The model under review builds one solid part; all positions refer to its coordinate system, in mm. A direction names the side the tool comes from. Coordinates: 2 decimals unless noted, no trailing zeros. Loops run counter-clockwise (first coordinate to the right, second up) from the corner with the lowest first, then second, coordinate; pieces in that order, holes last. Notation, with made-up numbers: M 59.25,-17 L 78.25,-17 A22 ccw 78.25,13 Z; hole C 16.25,36 d4. An arc over 180 degrees is marked long. Use CSV: the item, a comma, the result in double quotes. Start each with the question number.
1. Add section B-B, the plane x = 5.5. Write out the cut boundary in (y, z).
2. Add section A-A, the plane y = 3.5. Write out the cut boundary in (x, z).
3. Add section D-D, the plane x = 2.25. Write out the cut boundary in (y, z), then the cut area to 3 significant figures.
4. Add section C-C, the plane z = 0.25. Write out the cut boundary in (x, y).
5. Tool access review of faces 1 (the cylindrical face through (1.479, -3.859, 2.797)), 2 (the flat face through (0, 0, 0)), 3 (the flat face through (5.2, -2.5, -3)), 4 (the flat face through (5.2, -3, -3.5)), 5 (the flat face through (4, 4, 2)): name each direction out of +Z, -Z, +X, -X, +Y, -Y from which nothing blocks a thin tool from reaching the whole face with its end or side.
6. For L1, parallel to Z at x = 6.25, y = 2.5; L2, parallel to Z at x = 4.75, y = 3.5; L3, parallel to X at y = 1.5, z = 2, list the stretches that pass through material, from the lowest coordinate up.
7. Clearance check with flat-ended pins moving along their axes: P1, Ø1.3, axis at x = 6, y = 2, coming from the +Z side; P2, Ø1.1, axis at x = 6, y = -2.5, coming from the +Z side; P3, Ø1, axis at y = 3, z = 1, coming from the +X side. State where each tip first meets the part, or that it passes through.
from build123d import *

# Parameters (mm, degrees)
BOSS_EXTRUDE1_DEPTH = 3
BOSS_EXTRUDE2_DEPTH = 4.5
BOSS_EXTRUDE3_DEPTH = 3


with BuildPart() as part:
    # Sketch1 → Boss-Extrude1 (new body)
    with BuildSketch(Plane(origin=(0, 0, 0), x_dir=(0, 0, -1), z_dir=(1, 0, 0))):
        with BuildLine():
            Line((4, -5), (0, -5))
            ThreePointArc((0, -5), (-2.828427125, -3.828427125), (-4, -1))
            Line((-4, -1), (-4, 5))
            Line((-4, 5), (4, 5))
            Line((4, 5), (4, -5))
        make_face()
    extrude(amount=BOSS_EXTRUDE1_DEPTH)

    # Sketch2 → Boss-Extrude2 (add)
    with BuildSketch(Plane(origin=(3, 0, 0), x_dir=(0, 0, -1), z_dir=(1, 0, 0))):
        Polygon((4, -3), (4, 5), (2, 5), (2, -2), (3, -2), (3, -3), align=None)
    extrude(amount=BOSS_EXTRUDE2_DEPTH)

    # Sketch3 → Boss-Extrude3 (add)
    with BuildSketch(Plane(origin=(3, 0, 0), x_dir=(0, 0, -1), z_dir=(1, 0, 0))):
        with BuildLine():
            Line((2, 0), (2, 5))
            Line((2, 5), (-2, 5))
            Line((-2, 5), (-2, 3))
            ThreePointArc((-2, 3), (0.121320344, 2.121320344), (1, 0))
            Line((1, 0), (2, 0))
        make_face()
    extrude(amount=BOSS_EXTRUDE3_DEPTH)


solid = part.part
Computed:
1,outline,"M -3,-4 L 5,-4 L 5,2 L 3,2 A3 cw 0,-1 L 0,-2 L -2,-2 L -2,-3 L -3,-3 Z"
2,outline,"M 0,-4 L 7.5,-4 L 7.5,-2 L 6,-2 L 6,2 L 3,2 L 3,4 L 0,4 Z"
3,outline,"M -5,-4 L 5,-4 L 5,4 L -1,4 A4 ccw -5,0 Z"
3,area,"76.6 mm^2"
4,outline,"M 0,-4.99 L 3,-4.99 L 3,2.44 L 6,2.44 L 6,5 L 0,5 Z"
5,face 1,"+Z, +X, -X, -Y"
5,face 2,"+Z, -Z, -X, +Y, -Y"
5,face 3,"+Z, +X, -Y"
5,face 4,"+Z, -Z, +X, -Y"
5,face 5,"+Z, +X, +Y, -Y"
6,L1,"z = -4 to -2"
6,L2,"z = -4 to 2"
6,L3,"x = 0 to 3"
7,P1,"stops at z = 0.59"
7,P2,"stops at z = -2"
7,P3,"stops at x = 6"
